Geometry: final body of the model. Coordinates: model frame, mm. Round coordinates to 2 decimals unless told otherwise and drop trailing zeros. Loops run counter-clockwise (first coordinate to the right, second up) from the corner with the lowest first, then second, coordinate; pieces in that order, holes last. Notation, with made-up numbers: (50.5, -10) - (105.5, -10) arc R20 cw to (105.5, 4) - close; hole circle Ø8 at (54.25, -34.75). An arc over 180 degrees is marked (long way). Answer as a JSON object with one key per item and string values. Group by question number.
Item 1: Section B-B (y = 5.5). Return the cut outline in (x, z).
Item 2: Line query: line 1 (X direction, y = 15.5, z = 2); line 2 (Y direction, x = 10, z = 1.75); line 3 (Y direction, x = 10.5, z = 3.25). Output: solid intervals per line, ascending.
Item 3: Section C-C (y = 17). Return the cut outline in (x, z), plus the area to 3 significant figures.
Item 4: Draft query along Y for faces 1 (the face through (1.83, -9.23, 2.46)), 2 (the face through (-19.544, -1.66, 2.465)), 3 (the face through (-7, -5, 6.2)). Return one class per face: released by +Y, released by -Y, zero draft, split by the parting line, or undercut.
Item 5: Section A-A (x = 0). Return the cut outline in (y, z), plus the area to 3 significant figures.
Item 6: Section D-D (z = 3). Count the separate pieces of the cut face and the enclosed holes in it, plus the area to 3 significant figures.
Item 7: First-contact query: pin 1 (5 mm diameter, centred on x = -16, y = 16, fed in from +Z); pin 2 (8 mm diameter, centred on x = 10.5, y = 0.5, fed in from -Z); pin 3 (8 mm diameter, centred on x = -0.5, y = -0.5, fed in from +Z); pin 4 (1.5 mm diameter, centred on y = 14, z = 1.5, fed in from -X). Flat tips, straight axial feed; report the tip coordinate or a pass-through.
```python
from build123d import *

# Parameters (mm, degrees)
F0_R     = 25.4
F0_R_2   = 8.1
F2_DEPTH = 5
F1_R     = 8.05
F1_R_2   = 4.5
F3_DEPTH = 1
F1_R_3   = 9
F4_DEPTH = 6.2


with BuildPart() as f2:
    # F0 (on Top) → F2 (new body)
    with BuildSketch(Plane.XY):
        Circle(F0_R)
        with BuildLine():
            ThreePointArc((-4.606486482, -19.7909747686), (-5.9568852552, -18.7069483477), (-5.955029879, -16.9752767029))
            Line((-5.955029879, -16.9752767029), (-2.6440475771, -10.0999511093))
            ThreePointArc((-2.6440475771, -10.0999511093), (-1.8405240839, -9.2347532099), (-0.688998961, -8.9735879353))
            ThreePointArc((-0.688998961, -8.9735879353), (0, -9), (0.688998961, -8.9735879353))
            ThreePointArc((0.688998961, -8.9735879353), (1.8405240839, -9.2347532099), (2.6440475771, -10.0999511093))
            Line((2.6440475771, -10.0999511093), (5.955029879, -16.9752767029))
            ThreePointArc((5.955029879, -16.9752767029), (5.9568852552, -18.7069483477), (4.606486482, -19.7909747686))
            ThreePointArc((4.606486482, -19.7909747686), (0, -20.32), (-4.606486482, -19.7909747686))
        make_face(mode=Mode.SUBTRACT)
        with BuildLine():
            ThreePointArc((-18.3453044867, -8.7379747819), (-18.3397383666, -7.0063110887), (-16.9847061493, -5.9280820695))
            Line((-16.9847061493, -5.9280820695), (-9.5449964486, -4.230016879))
            ThreePointArc((-9.5449964486, -4.230016879), (-8.3675687887, -4.318794776), (-7.4454173842, -5.0562594846))
            ThreePointArc((-7.4454173842, -5.0562594846), (-7.0364833422, -5.6114082167), (-6.5862497328, -6.1336216428))
            ThreePointArc((-6.5862497328, -6.1336216428), (-6.0724727959, -7.1967541221), (-6.2479230487, -8.3644161528))
            Line((-6.2479230487, -8.3644161528), (-9.5589053506, -15.2397417464))
            ThreePointArc((-9.5589053506, -15.2397417464), (-10.9116239517, -16.3208719487), (-12.6011097989, -15.9409670922))
            ThreePointArc((-12.6011097989, -15.9409670922), (-15.8868157238, -12.6693127738), (-18.3453044867, -8.7379747819))
        make_face(mode=Mode.SUBTRACT)
        Circle(F0_R_2, mode=Mode.SUBTRACT)
        with BuildLine():
            ThreePointArc((12.6011097989, -15.9409670922), (10.9116239517, -16.3208719487), (9.5589053506, -15.2397417464))
            Line((9.5589053506, -15.2397417464), (6.2479230487, -8.3644161528))
            ThreePointArc((6.2479230487, -8.3644161528), (6.0724727959, -7.1967541221), (6.5862497328, -6.1336216428))
            ThreePointArc((6.5862497328, -6.1336216428), (7.0364833422, -5.6114082167), (7.4454173842, -5.0562594846))
            ThreePointArc((7.4454173842, -5.0562594846), (8.3675687887, -4.318794776), (9.5449964486, -4.230016879))
            Line((9.5449964486, -4.230016879), (16.9847061493, -5.9280820695))
            ThreePointArc((16.9847061493, -5.9280820695), (18.3397383666, -7.0063110887), (18.3453044867, -8.7379747819))
            ThreePointArc((18.3453044867, -8.7379747819), (15.8868157238, -12.6693127738), (12.6011097989, -15.9409670922))
        make_face(mode=Mode.SUBTRACT)
        with BuildLine():
            ThreePointArc((-18.269734037, 8.8948984378), (-16.9123944255, 9.9702213228), (-15.2245522643, 9.583079273))
            Line((-15.2245522643, 9.583079273), (-9.2583683118, 4.8252063378))
            ThreePointArc((-9.2583683118, 4.8252063378), (-8.5936635283, 3.8493042116), (-8.5952846582, 2.6685354869))
            ThreePointArc((-8.5952846582, 2.6685354869), (-8.7743512096, 2.0026884056), (-8.9019180428, 1.3250868497))
            ThreePointArc((-8.9019180428, 1.3250868497), (-9.4127738045, 0.2605476067), (-10.4350801844, -0.3303052303))
            Line((-10.4350801844, -0.3303052303), (-17.8747898851, -2.0283704208))
            ThreePointArc((-17.8747898851, -2.0283704208), (-19.5634577664, -1.6448460872), (-20.3198133854, -0.087086059))
            ThreePointArc((-20.3198133854, -0.087086059), (-19.8105351755, 4.521625378), (-18.269734037, 8.8948984378))
        make_face(mode=Mode.SUBTRACT)
        with BuildLine():
            ThreePointArc((-2, 10.246950766), (-2.3485543523, 9.1187986163), (-3.2727272727, 8.3838688085))
            ThreePointArc((-3.2727272727, 8.3838688085), (-3.9049536521, 8.1087198111), (-4.5142605006, 7.7859779176))
            ThreePointArc((-4.5142605006, 7.7859779176), (-5.6650641528, 7.5216516734), (-6.7644091044, 7.9525322677))
            Line((-6.7644091044, 7.9525322677), (-12.7305930568, 12.7104052029))
            ThreePointArc((-12.7305930568, 12.7104052029), (-13.4836088612, 14.2697824267), (-12.7372830441, 15.832372553))
            ThreePointArc((-12.7372830441, 15.832372553), (-8.8165175789, 18.3076873958), (-4.4366812227, 19.8297317109))
            ThreePointArc((-4.4366812227, 19.8297317109), (-2.749672532, 19.4389737228), (-2, 17.8779864638))
            Line((-2, 17.8779864638), (-2, 10.246950766))
        make_face(mode=Mode.SUBTRACT)
        with BuildLine():
            ThreePointArc((20.3198133854, -0.087086059), (19.5634577664, -1.6448460872), (17.8747898851, -2.0283704208))
            Line((17.8747898851, -2.0283704208), (10.4350801844, -0.3303052303))
            ThreePointArc((10.4350801844, -0.3303052303), (9.4127738045, 0.2605476067), (8.9019180428, 1.3250868497))
            ThreePointArc((8.9019180428, 1.3250868497), (8.7743512096, 2.0026884056), (8.5952846582, 2.6685354869))
            ThreePointArc((8.5952846582, 2.6685354869), (8.5936635283, 3.8493042116), (9.2583683118, 4.8252063378))
            Line((9.2583683118, 4.8252063378), (15.2245522643, 9.583079273))
            ThreePointArc((15.2245522643, 9.583079273), (16.9123944255, 9.9702213228), (18.269734037, 8.8948984378))
            ThreePointArc((18.269734037, 8.8948984378), (19.8105351755, 4.521625378), (20.3198133854, -0.087086059))
        make_face(mode=Mode.SUBTRACT)
        with BuildLine():
            Line((2, 10.246950766), (2, 17.8779864638))
            ThreePointArc((2, 17.8779864638), (2.749672532, 19.4389737228), (4.4366812227, 19.8297317109))
            ThreePointArc((4.4366812227, 19.8297317109), (8.8165175789, 18.3076873958), (12.7372830441, 15.832372553))
            ThreePointArc((12.7372830441, 15.832372553), (13.4836088612, 14.2697824267), (12.7305930568, 12.7104052029))
            Line((12.7305930568, 12.7104052029), (6.7644091044, 7.9525322677))
            ThreePointArc((6.7644091044, 7.9525322677), (5.6650641528, 7.5216516734), (4.5142605006, 7.7859779176))
            ThreePointArc((4.5142605006, 7.7859779176), (3.9049536521, 8.1087198111), (3.2727272727, 8.3838688085))
            ThreePointArc((3.2727272727, 8.3838688085), (2.3485543523, 9.1187986163), (2, 10.246950766))
        make_face(mode=Mode.SUBTRACT)
    extrude(amount=F2_DEPTH)



with BuildPart() as f3:
    # F1 (on face) → F3 (new body)
    with BuildSketch(Plane.XY):
        Circle(F1_R)
        Circle(F1_R_2, mode=Mode.SUBTRACT)
    extrude(amount=F3_DEPTH)


with BuildPart() as f2_1:
    add(f2.part)

    add(f3.part)  # F4 merges F3
    # F1 (on face) → F4 (join)
    with BuildSketch(Plane.XY):
        Circle(F1_R_3)
        Circle(F1_R, mode=Mode.SUBTRACT)
    extrude(amount=F4_DEPTH)


solid = f2_1.part
```
Values:
{
 "1": {"outline": "(-24.8, 0) - (-19.56, 0) - (-19.56, 5) - (-24.8, 5) - close; (-10.1, 0) - (10.1, 0) - (10.1, 5) - (7.12, 5) - (7.12, 6.2) - (5.88, 6.2) - (5.88, 1) - (-5.88, 1) - (-5.88, 6.2) - (-7.12, 6.2) - (-7.12, 5) - (-10.1, 5) - close; (19.56, 0) - (24.8, 0) - (24.8, 5) - (19.56, 5) - close"},
 "2": {"line 1": "x = -20.12 to -13.06, -2 to 2, 13.06 to 20.12", "line 2": "y = -23.35 to -15.84, -4.33 to -0.18, 5.42 to 10.53, 17.69 to 23.35", "line 3": "y = -23.13 to -16.18, -4.45 to -0.35, 5.82 to 10.93, 17.4 to 23.13"},
 "3": {"outline": "(-18.87, 0) - (-11.13, 0) - (-11.13, 5) - (-18.87, 5) - close; (-2, 0) - (2, 0) - (2, 5) - (-2, 5) - close; (11.13, 0) - (18.87, 0) - (18.87, 5) - (11.13, 5) - close", "area": "97.4 mm^2"},
 "4": {"face 1": "undercut", "face 2": "undercut", "face 3": "zero draft"},
 "5": {"outline": "(-25.4, 0) - (-20.32, 0) - (-20.32, 5) - (-25.4, 5) - close; (-9, 0) - (-4.5, 0) - (-4.5, 1) - (-8.05, 1) - (-8.05, 6.2) - (-9, 6.2) - close; (4.5, 0) - (25.4, 0) - (25.4, 5) - (9, 5) - (9, 6.2) - (8.05, 6.2) - (8.05, 1) - (4.5, 1) - close", "area": "126 mm^2"},
 "6": {"separate pieces": "1", "enclosed holes": "8", "area": "1,120 mm^2"},
 "7": {"pin 1": "stops at z = 5", "pin 2": "stops at z = 0", "pin 3": "stops at z = 1", "pin 4": "stops at x = -21.67"}
}
